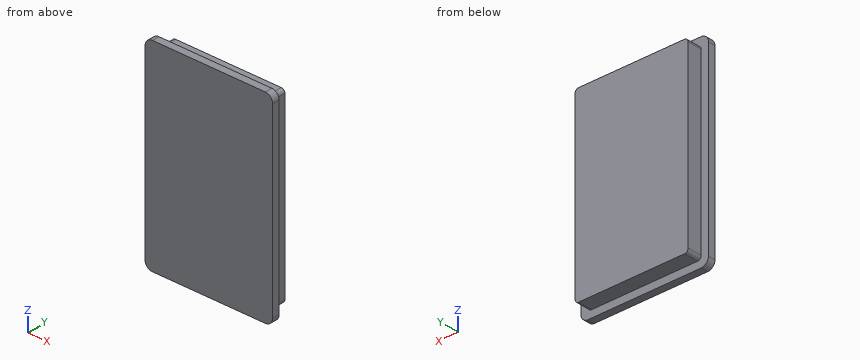
Autodesk Inventor part; units mm, degrees
ref_plane "YZ Plane" through (0, 0, 0) normal (1, 0, 0) x (0, 1, 0)
ref_plane "XZ Plane" through (0, 0, 0) normal (0, 1, 0) x (-1, 0, 0)
ref_plane "XY Plane" through (0, 0, 0) normal (0, 0, 1) x (1, 0, 0)
sketch "Sketch1" plane through (0, 0, 0) normal (0, 1, 0) x (-1, 0, 0)
  point P0 (0, 0)
sketch "Sketch2" plane through (0, 0, 0) normal (0, 1, 0) x (-1, 0, 0)
  line L0 (4.1714, 6.6076) -> (-13.3286, 6.6076)
  line L1 (-13.3286, 6.6076) -> (-13.3286, -20.8924)
  line L2 (-13.3286, -20.8924) -> (4.1714, -20.8924)
  line L3 (4.1714, -20.8924) -> (4.1714, 6.6076)
  point P0 (0, 0)
  dimension "d0" = 17.5
  dimension "d1" = 27.5
extrude "Extrusion1" add sketch "Sketch2" along normal blind 1
sketch "Sketch3" plane through (0, 1, 0) normal (0, 1, 0) x (1, 0, 0)
  line L0 (-4.1714, -6.6076) -> (13.3286, -6.6076)
  line L1 (-4.1714, -6.6076) -> (-3.1714, -6.6076)
  line L2 (-3.1714, -6.6076) -> (-3.1714, -5.6076)
  line L3 (-3.1714, -5.6076) -> (12.3286, -5.6076)
  line L4 (12.3286, -5.6076) -> (12.3286, 19.8924)
  line L5 (12.3286, 19.8924) -> (-3.1714, 19.8924)
  line L6 (-3.1714, 19.8924) -> (-3.1714, -5.6076)
  point P0 (0, 0)
  dimension "d4" = 1
  dimension "d5" = 1
  dimension "d6" = 15.5
  dimension "d7" = 25.5
extrude "Extrusion2" add sketch "Sketch3" along normal blind 2
fillet "Fillet1" radius 1 4 edges at (-4.1714, 0.5, -20.8924) (-4.1714, 0.5, 6.6076) (13.3286, 0.5, 6.6076) (13.3286, 0.5, -20.8924)
fillet "Fillet2" radius 0.5 4 edges at (12.3286, 2, -19.8924) (12.3286, 2, 5.6076) (-3.1714, 2, -19.8924) (-3.1714, 2, 5.6076)
properties part number "plug"
Input: part model. Units: mm. Frame: model coordinates. Coordinates: 2 decimals unless noted, no trailing zeros. Loops run counter-clockwise (first coordinate to the right, second up) from the corner with the lowest first, then second, coordinate; pieces in that order, holes last. Notation, with made-up numbers: (14, -17.75) -> (27, -17.75) arc R25 ccw to (27, 5.25) -> close; hole circle Ø7 at (1, -35.75). An arc over 180 degrees is marked (long way). Write item = value, one per line. Start each with the question number.
Item 1: Cut plane A-A, the plane z = -13. Return loops of the section in (x, y), plus the area to 3 significant figures.
Item 2: Cut plane B-B, the plane x = 4. Return loops of the section in (y, z).
Item 3: First-contact query: P1, Ø1.6, axis at x = 1.5, y = 2, coming from the +Z side; P2, Ø0.6, axis at y = 2.5, z = -12, coming from the +X side; P3, Ø1.6, axis at y = 2, z = -2, coming from the -X side. Flat tips, straight axial feed; report the tip coordinate or a pass-through.
Item 4: Material intervals for line 1 (Z direction, x = 0.5, y = 2.5); line 2 (Y direction, x = 12.75, z = -13.75); line 3 (X direction, y = 1.45, z = -17), sorted ascending.
Ans:
q1.outline = (-4.17, 0) -> (13.33, 0) -> (13.33, 1) -> (12.33, 1) -> (12.33, 3) -> (-3.17, 3) -> (-3.17, 1) -> (-4.17, 1) -> close
q1.area = 48.5 mm²
q2.outline = (0, -20.89) -> (1, -20.89) -> (1, -19.89) -> (3, -19.89) -> (3, 5.61) -> (1, 5.61) -> (1, 6.61) -> (0, 6.61) -> close
q3.P1 = 5.61
q3.P2 = 12.33
q3.P3 = -3.17
q4.line_1 = -19.89 to 5.61
q4.line_2 = 0 to 1
q4.line_3 = -3.17 to 12.33
